from build123d import *

# Parameters (mm, degrees)
SKETCH1_R           = 2.7
BOSS_EXTRUDE1_DEPTH = 3
SKETCH2_R           = 1.696293742
BOSS_EXTRUDE2_DEPTH = 6
CUT_EXTRUDE1_DEPTH  = 2


with BuildPart() as part:
    # Sketch1 → Boss-Extrude1 (new body)
    with BuildSketch(Plane(origin=(0, 0, 0), x_dir=(1, 0, 0), z_dir=(0, 1, 0))):
        with Locations((184.714490272, -125.24429514)):
            Circle(SKETCH1_R)
    extrude(amount=-BOSS_EXTRUDE1_DEPTH)

    # Sketch2 → Boss-Extrude2 (add)
    with BuildSketch(Plane.XZ.offset(3)):
        with Locations((184.714490272, 125.24429514)):
            Circle(SKETCH2_R)
    extrude(amount=BOSS_EXTRUDE2_DEPTH)

    # Sketch3 → Cut-Extrude1 (cut)
    with BuildSketch(Plane(origin=(0, 0, 0), x_dir=(1, 0, 0), z_dir=(0, 1, 0))):
        Polygon((184.714490272, -123.800919467), (183.464490272, -124.522607304), (183.464490272, -125.965982977), (184.714490272, -126.687670813), (185.964490272, -125.965982977), (185.964490272, -124.522607304), align=None)
    extrude(amount=-CUT_EXTRUDE1_DEPTH, mode=Mode.SUBTRACT)


solid = part.part
Source: CAD feature listing. Evaluate the final solid. Frame: model axes, mm. A direction names the side the tool comes from. Give positions to 0.01 mm unless a question says otherwise; leave off trailing zeros. Write each loop counter-clockwise with the first axis right and the second up, starting at its lowest first coordinate (ties: lowest second). Pieces come first, ordered by that corner, then holes. Notation, with made-up numbers: M 4.25,76.5 L 22.25,76.5 A20 cw 22.25,111.5 Z; hole C -24,12 d10. An arc over 180 degrees is marked long. Return JSON: item names as keys, results as strings. Group by question number.
1) Cut plane A-A, the plane x = 185.3. Output: boundary loops of the cut face in (y, z).
2) Cut plane C-C, the plane z = 123.9. Output: boundary loops of the cut face in (x, y), then the cut area to 3 significant figures.
3) Cut plane D-D, the plane x = 186.25. Output: boundary loops of the cut face in (y, z).
4) Cut plane B-B, the plane y = -1.75. Output: boundary loops of the cut face in (x, z).
5) Draft query along X for faces 4 (the face through (185.964, -1, 125)), 5 (the face through (185, -9, 125)), 6 (the face through (183.37, -5.96, 124.21)). Return one class per face: released by +X, released by -X, zero draft, split by the parting line, or undercut.
6) Set-up query: faces 1 (the face through (183, -3, 126)), 2 (the face through (184.098, -0.986, 124.157)), 3 (the face through (182.017, -1.479, 125.126)). Return all of +Z, -Z, +X, -X, +Y, -Y with unobstructed straight access to the full face (end or side cutting, diameter ignored); none if empty.
7) Ray query, L1, parallel to Y at x = 184.3, z = 125.5; L2, parallel to X at y = -1.5, z = 124.2; L3, parallel to X at y = -6.5, z = 125.2. Return the intervals inside material, ascending.
Data:
{
 "1": {"outline": "M -9,123.65 L -3,123.65 L -3,122.61 L 0,122.61 L 0,124.14 L -2,124.14 L -2,126.35 L 0,126.35 L 0,127.88 L -3,127.88 L -3,126.84 L -9,126.84 Z"},
 "2": {"outline": "M 182.37,-3 L 183.68,-3 L 183.68,-9 L 185.75,-9 L 185.75,-3 L 187.06,-3 L 187.06,0 L 184.89,0 L 184.89,-2 L 184.54,-2 L 184.54,0 L 182.37,0 Z", "area": "25.8 mm²"},
 "3": {"outline": "M -9,124.52 L -3,124.52 L -3,123.02 L 0,123.02 L 0,127.47 L -3,127.47 L -3,125.97 L -9,125.97 Z"},
 "4": {"outline": "C 184.71,125.24 d5.4; hole M 183.46,124.52 L 184.71,123.8 L 185.96,124.52 L 185.96,125.97 L 184.71,126.69 L 183.46,125.97 Z"},
 "5": {"face 4": "undercut", "face 5": "zero draft", "face 6": "split by the parting line"},
 "6": {"face 1": "-Y", "face 2": "+Y", "face 3": "+Y, -Y"},
 "7": {"L1": "y = -9 to -2", "L2": "x = 182.22 to 184.02, 185.41 to 187.2", "L3": "x = 183.02 to 186.41"}
}
